For this review, take the finished solid that the model builds, in its own axes (mm). A direction names the side the tool comes from. Give positions to 0.01 mm unless a question says otherwise; leave off trailing zeros. Order: outer loops, then holes, each group sorted by start corner. A loop starts at its lowest first (then second) coordinate and runs counter-clockwise, first axis right, second up.
Item 1: Consider section D-D (x = -8.5). Give the boundary of the cut face in (y, z).
Item 2: The part is to be moulded in two halves that separate along Y. For faces 1 (the flat face through (20, 19, 19)), 2 (the cylindrical face through (-2.38, -10.74, 38.99)), 3 (the cylindrical face through (-17, 15.57, 35.78)), say which applies: released by +Y, released by -Y, zero draft, split by the parting line, or undercut.
Item 3: Machinability: for faces 4 (the flat face through (-19, -20, 19)), 5 (the flat face through (-16, 16, 33.5)), which of the approach directions +Z, -Z, +X, -X, +Y, -Y give a long, thin tool a straight path to every point of the face, cutting with its end or side? Answer none if there is none.
Item 4: Consider section A-A (x = 15.5). Give the boundary of the cut face in (y, z), plus the area to 3 significant figures.
Item 5: For probe 1 along Y at (x, z) = (15.5, 34.45); probe 2 along Z at (x, y) = (-5.5, 17); probe 3 along Z at (x, y) = (-6, 7), list the stretches that pass through material, from the lowest coordinate up.
Item 6: For P1, Ø1, axis at x = 11, y = -13, coming from the +Z side; P2, Ø1.5, axis at x = -15.5, y = -15.5, coming from the +Z side; P3, Ø4, axis at x = -15.5, y = -15.5, coming from the -Z side, all flat-tipped, find the tip position at first contact; note any pin that passes through.
Item 7: Consider section C-C (z = 55). Give the boundary of the cut face in (x, y).
```python
from build123d import *

# Parameters (mm, degrees)
SKETCH1_W           = 42
SKETCH1_H           = 42
BOSS_EXTRUDE1_DEPTH = 38
SKETCH2_R           = 11
BOSS_EXTRUDE2_DEPTH = 2
SKETCH3_R           = 2.5
BOSS_EXTRUDE3_DEPTH = 21.5
SKETCH4_R           = 1.5
CUT_EXTRUDE1_DEPTH  = 4.5
CHAMFER1_SIZE       = 3


with BuildPart() as part:
    # Sketch1 → Boss-Extrude1 (new body)
    with BuildSketch(Plane.XY):
        Rectangle(SKETCH1_W, SKETCH1_H)
    extrude(amount=BOSS_EXTRUDE1_DEPTH)

    # Sketch2 → Boss-Extrude2 (add)
    with BuildSketch(Plane.XY.offset(38)):
        Circle(SKETCH2_R)
    extrude(amount=BOSS_EXTRUDE2_DEPTH)

    # Sketch3 → Boss-Extrude3 (add)
    with BuildSketch(Plane.XY.offset(40)):
        Circle(SKETCH3_R)
    extrude(amount=BOSS_EXTRUDE3_DEPTH)

    # Sketch4 → Cut-Extrude1 (cut)
    with BuildSketch(Plane.XY.offset(38)):
        with Locations((15.5, 15.5)):
            Circle(SKETCH4_R)
        with Locations((15.5, -15.5)):
            Circle(SKETCH4_R)
        with Locations((-15.5, -15.5)):
            Circle(SKETCH4_R)
        with Locations((-15.5, 15.5)):
            Circle(SKETCH4_R)
    extrude(amount=-CUT_EXTRUDE1_DEPTH, mode=Mode.SUBTRACT)

    # Chamfer1
    chamfer1_edges = [part.edges().sort_by_distance(p)[0] for p in [
        (21, -21, 19),
        (-21, -21, 19),
        (-21, 21, 19),
        (21, 21, 19),
    ]]
    chamfer(chamfer1_edges, length=CHAMFER1_SIZE)


solid = part.part
```
Resolved:
1. outline: (-21, 0) - (21, 0) - (21, 38) - (6.98, 38) - (6.98, 40) - (-6.98, 40) - (-6.98, 38) - (-21, 38) - close
2. face 1: released by +Y
2. face 2: split by the parting line
2. face 3: undercut
3. face 4: +Z, -Z, -X, -Y
3. face 5: +Z
4. outline: (-21, 0) - (21, 0) - (21, 38) - (17, 38) - (17, 33.5) - (14, 33.5) - (14, 38) - (-14, 38) - (-14, 33.5) - (-17, 33.5) - (-17, 38) - (-21, 38) - close
4. area: 1,570 mm2
5. probe 1: y = -21 to -17, -14 to 14, 17 to 21
5. probe 2: z = 0 to 38
5. probe 3: z = 0 to 40
6. P1: stops at z = 38
6. P2: stops at z = 33.5
6. P3: stops at z = 0
7. outline: circle Ø5 at (0, 0)
